from build123d import *

# Parameters (mm, degrees)
CORTE_EXTRUS_O1_DEPTH = 4


with BuildPart() as part:
    # Esboço1 → Revolução1 (revolve)
    with BuildSketch(Plane.XY):
        with BuildLine():
            Line((0, 0), (6, 0))
            Line((6, 0), (6, 20))
            Line((6, 20), (10.5, 20))
            Line((10.5, 20), (10.5, 20.8))
            ThreePointArc((10.5, 20.8), (8.962310601, 24.512310601), (5.25, 26.05))
            Line((5.25, 26.05), (0, 26.05))
            Line((0, 26.05), (0, 0))
        make_face()
    revolve(axis=Axis((0, 26.05, 0), (0, -1, 0)))

    # Esboço2 → Corte-extrusão1 (cut)
    with BuildSketch(Plane(origin=(0, 26.05, 0), x_dir=(1, 0, 0), z_dir=(0, 1, 0))):
        Polygon((-4, -2.309401077), (0, -4.618802154), (4, -2.309401077), (4, 2.309401077), (0, 4.618802154), (-4, 2.309401077), align=None)
    extrude(amount=-CORTE_EXTRUS_O1_DEPTH, mode=Mode.SUBTRACT)


solid = part.part
Verification items for the finished model (mm, model axes). A direction names the side the tool comes from. Give positions to 0.01 mm unless a question says otherwise; leave off trailing zeros. Order: outer loops, then holes, each group sorted by start corner. A loop starts at its lowest first (then second) coordinate and runs counter-clockwise, first axis right, second up. Notation, with made-up numbers: M 57.25,51 L 99.25,51 A9 cw 99.25,57 Z; hole C -11.75,84 d10. An arc over 180 degrees is marked long. Answer as a JSON object with one key per item and string values. Group by question number.
1) Mould release check, pull along Z, two halves, no side actions. Record for faces 1 (the face through (-4, 24, 0)), 2 (the face through (2, 26.05, -4)), 3 (the face through (10, 20.4, 3.2)): released by +Z, released by -Z, zero draft, split by the parting line, or undercut.
2) Cross-section at A-A (y = 10.25). Enter the section's corners in (x, z).
3) Depth check by flat-ended pin: pin 1 Ø1 at (y, z) = (9, 2.5) entering from +X; pin 2 Ø4 at (y, z) = (9.5, -3) entering from -X; pin 3 Ø5 at (x, z) = (-6, -1.5) entering from +Y; pin 4 Ø3 at (x, z) = (-8, -5.5) entering from -Y. Enter the tip coordinate at first touch or a pass-through.
4) Access from +Z, -Z, +X, -X, +Y, -Y to the whole of each face (thin tool, end or side, straight path). Record for faces 4 (the face through (0, 0, 0)), 5 (the face through (-6, 10, 0)), 6 (the face through (0, 22.05, 0)).
5) Scan lines: line 1 along Y through (x, z) = (0.25, 2.75); line 2 along X through (y, z) = (3, -0.25); line 3 along Y through (x, z) = (-1.5, -5.25). Record each from-to range of solid material in increasing order. Write a range as [from, to].
Result sheet:
{
 "1": {"face 1": "undercut", "face 2": "zero draft", "face 3": "split by the parting line"},
 "2": {"outline": "C 0,0 d12"},
 "3": {"pin 1": "stops at x = 5.66", "pin 2": "stops at x = -5.92", "pin 3": "stops at y = 26.05", "pin 4": "stops at y = 20"},
 "4": {"face 4": "+Z, -Z, +X, -X, -Y", "face 5": "-Y", "face 6": "+Y"},
 "5": {"line 1": "y = [0, 22.05]", "line 2": "x = [-5.99, 5.99]", "line 3": "y = [0, 26.05]"}
}
